Design review of the part built by this model. Coordinates are the model's own, in mm. Face numbers are marked on the shaded views. A direction names the side the tool comes from. Coordinates: 2 decimals unless noted, no trailing zeros. Write each loop counter-clockwise with the first axis right and the second up, starting at its lowest first coordinate (ties: lowest second). Pieces come first, ordered by that corner, then holes. Notation, with made-up numbers: (80, 2.5) - (128, 2.5) arc R22 cw to (128, 12.5) - close; hole circle Ø1 at (-4, 77). An arc over 180 degrees is marked (long way). One line per item, written item: value.
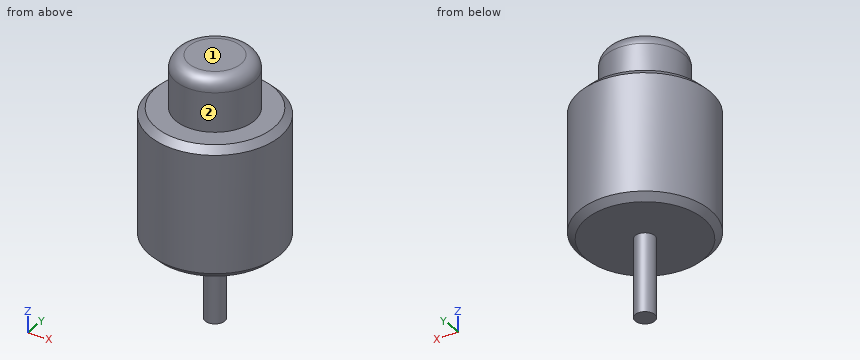
Autodesk Inventor part; units mm, degrees
ref_plane "YZ Plane" through (0, 0, 0) normal (1, 0, 0) x (0, 1, 0)
ref_plane "XZ Plane" through (0, 0, 0) normal (0, 1, 0) x (-1, 0, 0)
ref_plane "XY Plane" through (0, 0, 0) normal (0, 0, 1) x (1, 0, 0)
sketch "Sketch1" plane through (0, 0, 0) normal (0, 0, 1) x (1, 0, 0)
  circle A0 centre (0, 0) radius 2.5
  dimension "d0" = 5
extrude "Extrusion1" add sketch "Sketch1" along normal blind 5
chamfer "Chamfer1" distance 0.25 angle 45 2 edges at (-2.5, 0, 5) (-2.5, 0, 0)
sketch "Sketch2" plane through (0, 0, 5) normal (0, 0, 1) x (1, 0, 0)
  circle A0 centre (0, 0) radius 1.5
  dimension "d12" = 3
extrude "Extrusion2" add sketch "Sketch2" along normal blind 2
fillet "Fillet1" radius 0.5 1 edges at (-1.5, 0, 7)
sketch "Sketch3" plane through (0, 0, 0) normal (0, 0, -1) x (-1, 0, 0)
  circle A0 centre (0, 0) radius 0.375
  dimension "d9" = 0.75
extrude "Extrusion3" add sketch "Sketch3" along normal blind 3
properties part number "DC motor_CPY1"
1. Consider section C-C, the plane z = 6.25. Write out the cut boundary in (x, y).
Answer block:
outline: circle Ø3 at (0, 0)
2. Insertion check: pin 1 Ø1.5 at (x, z) = (-1.5, 0) entering from -Y. The pin has a flat end and moves straight along its axis. Give the tip position at first contact, or say it passes through.
Answer block:
pin 1: stops at y = -2.37
3. For the marked faces 1 and 2, list the 3-axis set-ups (+Z, -Z, +X, -X, +Y, -Y) from which the entire face can be reached by the end or side of a thin tool; tool diameter is ignored.
Answer block:
face 1: +Z, +X, -X, +Y, -Y
face 2: +Z
4. Wall thickness on line 1 along Z through (x, y) = (-1.1, -1.95); line 2 along Z through (x, y) = (0.85, -0.8); line 3 along X through (y, z) = (-0.85, 5.75): over which ranges is each line inside the solid? List them lowest first.
Answer block:
line 1: z = 0 to 5
line 2: z = 0 to 6.97
line 3: x = -1.24 to 1.24
5. Consider section D-D, the plane z = -2. Write out the cut boundary in (x, y) (3 decimals).
Answer block:
outline: circle Ø0.75 at (0, 0)
6. Consider section A-A, the plane y = 0. Write out the cut boundary in (x, z) (3 decimals), then the cut area to 3 significant figures.
Answer block:
outline: (-2.5, 0.25) - (-2.25, 0) - (-0.375, 0) - (-0.375, -3) - (0.375, -3) - (0.375, 0) - (2.25, 0) - (2.5, 0.25) - (2.5, 4.75) - (2.25, 5) - (1.5, 5) - (1.5, 6.5) arc R0.5 ccw to (1, 7) - (-1, 7) arc R0.5 ccw to (-1.5, 6.5) - (-1.5, 5) - (-2.25, 5) - (-2.5, 4.75) - close
area: 33.0 mm^2
